```python
from build123d import *

# Parameters (mm, degrees)
BOSS_EXTRUDE1_DEPTH = 9.525
FILLET1_R           = 8.255
FILLET3_R           = 10.795
SKETCH2_R           = 3.175
CUT_EXTRUDE1_DEPTH  = 122.954832076
SKETCH3_R           = 3.175
SKETCH3_R_2         = 2.38125
CUT_EXTRUDE2_DEPTH  = 122.954832076


with BuildPart() as part:
    # Sketch1 → Boss-Extrude1 (new body)
    with BuildSketch(Plane.XY):
        with BuildLine():
            Line((12.7, 57.15), (-12.7, 57.15))
            ThreePointArc((-12.7, 57.15), (-71.390768363, 60.032513664), (-101.6, 9.630951188))
            Line((-101.6, 9.630951188), (-85.725, 9.630951188))
            ThreePointArc((-85.725, 9.630951188), (-58.470420375, 48.45173734), (-12.7, 36.004481953))
            Line((-12.7, 36.004481953), (-12.7, -57.15))
            Line((-12.7, -57.15), (12.7, -57.15))
            Line((12.7, -57.15), (12.7, 57.15))
        make_face()
    extrude(amount=BOSS_EXTRUDE1_DEPTH)

    # Fillet1
    fillet1_edges = [part.edges().sort_by_distance(p)[0] for p in [
        (-12.7, 36.004481953, 4.7625),
    ]]
    fillet(fillet1_edges, radius=FILLET1_R)

    # Chamfer1
    # the kernel refuses this chamfer: 16.925734726, 15.24 mm, written as the material it takes off along each edge
    with BuildSketch(Plane(origin=(-85.725, 9.630951188, -32.922584323), x_dir=(0.18505799374320953, 0.982727601602671, 0), z_dir=(0, 0, 1))) as chamfer1_piece_1:
        with BuildLine():
            Line((13.024984464, 0), (-2.866629235, 12.853244189))
            Line((-2.866629235, 12.853244189), (-3.199296969, 12.790599339))
            ThreePointArc((-3.199296969, 12.790599339), (-1.550509453, 6.404553068), (-0.332667734, -0.06264485))
            Line((-0.332667734, -0.06264485), (0.06264485, -0.332667734))
            ThreePointArc((0.06264485, -0.332667734), (6.502538231, 0.358645822), (12.985122864, -0.336159562))
            Line((12.985122864, -0.336159562), (13.024984464, 0))
        make_face()
    extrude(amount=75.370168646, mode=Mode.SUBTRACT)

    # Fillet3
    fillet3_edges = [part.edges().sort_by_distance(p)[0] for p in [
        (-12.7, 57.15, 4.7625),
        (12.7, 57.15, 4.7625),
    ]]
    fillet(fillet3_edges, radius=FILLET3_R)

    # Sketch2 → Cut-Extrude1 (cut, through all)
    with BuildSketch(Plane.XY.offset(9.525)):
        with Locations((0, -50.8)):
            Circle(SKETCH2_R)
        with Locations((0, -38.1)):
            Circle(SKETCH2_R)
    extrude(amount=-CUT_EXTRUDE1_DEPTH, mode=Mode.SUBTRACT)

    # Sketch3 → Cut-Extrude2 (cut, through all)
    with BuildSketch(Plane.XY.offset(9.525)):
        with Locations((0, -12.7)):
            Circle(SKETCH3_R)
        with Locations((0, 44.45)):
            Circle(SKETCH3_R)
        with Locations((-91.600885684, 25.42155909)):
            Circle(SKETCH3_R_2)
        with Locations((-78.380902496, 45.979860037)):
            Circle(SKETCH3_R_2)
        with Locations((-58.239749026, 57.405339102)):
            Circle(SKETCH3_R_2)
        with Locations((-32.074025979, 57.790940658)):
            Circle(SKETCH3_R_2)
    extrude(amount=-CUT_EXTRUDE2_DEPTH, mode=Mode.SUBTRACT)


solid = part.part
```
Input: part model. Units: mm. Frame: model coordinates. A direction names the side the tool comes from. Round coordinates to 2 decimals unless told otherwise and drop trailing zeros. Order: outer loops, then holes, each group sorted by start corner. A loop starts at its lowest first (then second) coordinate and runs counter-clockwise, first axis right, second up. Notation, with made-up numbers: (-23.75, -22) - (17.25, -22) arc R27 ccw to (17.25, 1) - close; hole circle Ø9 at (84, -13.5). An arc over 180 degrees is marked (long way). One line per question, with ' | ' between items. Start each with the question number.
1) Cut plane A-A, the plane x = 0. Return the cut outline in (y, z) (3 decimals).
2) Cut plane B-B, the plane y = -12.7. Return the cut outline in (x, z) (3 decimals).
3) Set-up query: faces 4 (the cylindrical face through (-34.453, 57.896, 4.829)), 5 (the flat face through (-100, 9.631, 5)), 6 (the flat face through (-90.999, 15.898, 4.696)). Return all of +Z, -Z, +X, -X, +Y, -Y with unobstructed straight access to the full face (end or side cutting, diameter ignored); none if empty.
4) Pull-direction query (Y, two-part tool) for faces 1 (the flat face through (-4, 57.15, 5)), 2 (the cylindrical face through (1.707, -35.423, 4.829)), 3 (the cylindrical face through (-54.737, 49.603, 4.696)); classes: +Y half, -Y half, draft (parallel to the pull), parting line (faces both ways), or undercut.
5) Ray query, probe 1 along X at (y, z) = (47, 3.25); probe 2 along X at (y, z) = (-6.5, 8.5); probe 3 along X at (y, z) = (30.5, 4.25). Return the intervals inside material, ascending.
6) Cut plane C-C, the plane z = 1.5. Give the number of separate pieces and of enclosed holes in the cut face, then the cut area to 3 significant figures.
7) Cut plane D-D, the plane y = 18.5. Return the cut outline in (x, z) (1 decimal), then the cut area to 3 significant figures.
8) Contact query for flat-ended pins moving along their axis: P1, Ø3, axis at x = -32.07, y = 57.79, coming from the +Z side; P2, Ø1.5, axis at x = -73.5, z = 1.5, coming from the -Y side; P3, Ø2, axis at y = 22, z = 4.5, coming from the -X side; P4, Ø5, axis at x = -5, z = 3, coming from the +Y side. Output: stop coordinate, or through.
Worked out:
1) outline: (-57.15, 0) - (-53.975, 0) - (-53.975, 9.525) - (-57.15, 9.525) - close; (-47.625, 0) - (-41.275, 0) - (-41.275, 9.525) - (-47.625, 9.525) - close; (-34.925, 0) - (-15.875, 0) - (-15.875, 9.525) - (-34.925, 9.525) - close; (-9.525, 0) - (41.275, 0) - (41.275, 9.525) - (-9.525, 9.525) - close; (47.625, 0) - (57.15, 0) - (57.15, 9.525) - (47.625, 9.525) - close
2) outline: (-12.7, 0) - (-3.175, 0) - (-3.175, 9.525) - (-12.7, 9.525) - close; (3.175, 0) - (12.7, 0) - (12.7, 9.525) - (3.175, 9.525) - close
3) face 4: +Z, -Z | face 5: +Z, -Z, -X, -Y | face 6: +Z, -Z, -Y
4) face 1: +Y half | face 2: undercut | face 3: -Y half
5) probe 1: x = -87.69 to -80.53, -76.23 to -61.98, -26.92 to -1.89, 1.89 to 12.68 | probe 2: x = -12.7 to 12.7 | probe 3: x = -97.65 to -80.06, -12.7 to 12.7
6) separate pieces: 1 | enclosed holes: 8 | area: 4,390 mm^2
7) outline: (-100.9, 0) - (-87.9, 0) - (-87.9, 9.5) - (-100.9, 9.5) - close; (-12.7, 0) - (12.7, 0) - (12.7, 9.5) - (-12.7, 9.5) - close | area: 365 mm^2
8) P1: passes through | P2: stops at y = 38.19 | P3: stops at x = -100.46 | P4: stops at y = 57.15
